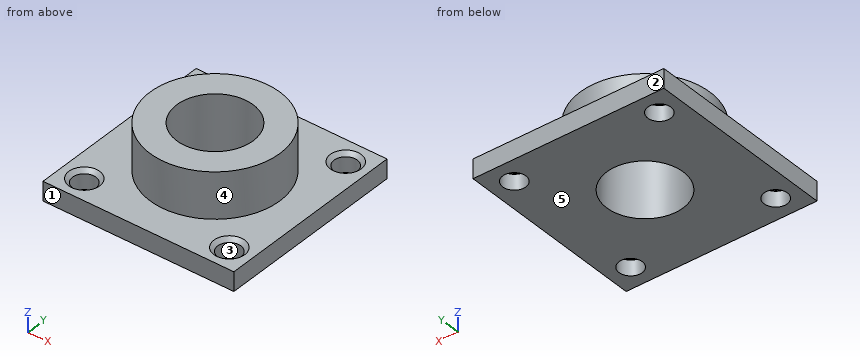
```python
from build123d import *

# Parameters (mm, degrees)
F0_W     = 254
F0_H     = 254
F0_R     = 50.8
F1_DEPTH = 25.4
F2_R     = 86.3600000739
F2_R_2   = 50.8
F3_DEPTH = 60.96
F4_R     = 15.431866001
F5_DEPTH = 162.56
F6_SIZE  = 5.08


with BuildPart() as f1:
    # F0 (on Top) → F1 (new body)
    with BuildSketch(Plane.XY):
        Rectangle(F0_W, F0_H)
        Circle(F0_R, mode=Mode.SUBTRACT)
    extrude(amount=F1_DEPTH)

    # F2 (on face) → F3 (join)
    with BuildSketch(Plane.XY.offset(25.4)):
        Circle(F2_R)
        Circle(F2_R_2, mode=Mode.SUBTRACT)
    extrude(amount=F3_DEPTH)

    # F4 (on face) → F5 (cut)
    with BuildSketch(Plane(origin=(0, 0, 0), x_dir=(1, 0, 0), z_dir=(0, 0, -1))):
        with Locations((-96.5199992061, -96.5199992061)):
            Circle(F4_R)
        with Locations((96.5199992061, -96.5199992061)):
            Circle(F4_R)
        with Locations((96.5199992061, 96.5199992061)):
            Circle(F4_R)
        with Locations((-96.5199992061, 96.5199992061)):
            Circle(F4_R)
    extrude(amount=-F5_DEPTH, mode=Mode.SUBTRACT)

    # F6
    f6_edges = [f1.edges().sort_by_distance(p)[0] for p in [
        (-111.951865, 96.519999, 25.4),
        (81.088133, 96.519999, 25.4),
        (81.088133, -96.519999, 25.4),
        (-111.951865, -96.519999, 25.4),
    ]]
    chamfer(f6_edges, length=F6_SIZE)


solid = f1.part
```
Geometry: final body of the model. Coordinates: model frame, mm. Face numbers are marked on the shaded views. A direction names the side the tool comes from. Coordinates: 2 decimals unless noted, no trailing zeros. Order: outer loops, then holes, each group sorted by start corner. A loop starts at its lowest first (then second) coordinate and runs counter-clockwise, first axis right, second up. Notation, with made-up numbers: (82, 6.25) -> (134, 6.25) arc R23 ccw to (134, 45.25) -> close; hole circle Ø10 at (-24, 67). An arc over 180 degrees is marked (long way). Write item = value, one per line.
(1) Cut plane B-B on y = 0. Return loops of the section in (x, z).
Solved:
outline = (-127, 0) -> (-50.8, 0) -> (-50.8, 86.36) -> (-86.36, 86.36) -> (-86.36, 25.4) -> (-127, 25.4) -> close; (50.8, 0) -> (127, 0) -> (127, 25.4) -> (86.36, 25.4) -> (86.36, 86.36) -> (50.8, 86.36) -> close
(2) Cut plane A-A on x = -12.5. Return loops of the section in (y, z).
Solved:
outline = (-127, 0) -> (-49.24, 0) -> (-49.24, 86.36) -> (-85.45, 86.36) -> (-85.45, 25.4) -> (-127, 25.4) -> close; (49.24, 0) -> (127, 0) -> (127, 25.4) -> (85.45, 25.4) -> (85.45, 86.36) -> (49.24, 86.36) -> close
(3) Pin query (flat end, axial travel): pin 1 Ø3 at (y, z) = (9.5, 65.5) entering from +X; pin 2 Ø10 at (x, z) = (13, 69) entering from -Y; pin 3 Ø8 at (y, z) = (3.5, 58.5) entering from -X; pin 4 Ø24.5 at (x, y) = (96.52, 96.52) entering from +Z. Return the tip coordinate at first contact, or that it passes through.
Solved:
pin_1 = 85.99
pin_2 = -85.99
pin_3 = -86.36
pin_4 = through
(4) Cut plane C-C on z = 17. Return loops of the section in (x, y).
Solved:
outline = (-127, -127) -> (127, -127) -> (127, 127) -> (-127, 127) -> close; hole circle Ø30.86 at (-96.52, -96.52); hole circle Ø30.86 at (-96.52, 96.52); hole circle Ø101.6 at (0, 0); hole circle Ø30.86 at (96.52, -96.52); hole circle Ø30.86 at (96.52, 96.52)
(5) Line query: line 1 (Y direction, x = 96, z = 5); line 2 (Y direction, x = 96.52, z = 14.5). Output: solid intervals per line, ascending.
Solved:
line_1 = -127 to -111.94, -81.1 to 81.1, 111.94 to 127
line_2 = -127 to -111.95, -81.09 to 81.09, 111.95 to 127
(6) Pull-direction query (Y, two-part tool) for the marked faces 1, 2 and 3; classes: pulls with the +Y half, pulls with the -Y half, needs draft (parallel to the pull), parting line crosses it, or undercut.
Solved:
face_1 = pulls with the -Y half
face_2 = pulls with the +Y half
face_3 = undercut
(7) Cut plane D-D on z = 39. Return loops of the section in (x, y).
Solved:
outline = circle Ø172.72 at (0, 0); hole circle Ø101.6 at (0, 0)
(8) Access query for the marked faces 4 and 5. Directions: +Z, -Z, +X, -X, +Y, -Y. A direction counts if a zero-diameter tool reaches every point of the face in a straight line with its end or side. Return the directions, or none.
Solved:
face_4 = +Z
face_5 = -Z, +X, -X, +Y, -Y
